Autodesk Inventor part; units mm, degrees
ref_plane "YZ Plane" through (0, 0, 0) normal (1, 0, 0) x (0, 1, 0)
ref_plane "XZ Plane" through (0, 0, 0) normal (0, 1, 0) x (-1, 0, 0)
ref_plane "XY Plane" through (0, 0, 0) normal (0, 0, 1) x (1, 0, 0)
sketch "Sketch1" plane through (0, 0, 0) normal (0, 1, 0) x (-1, 0, 0)
  line L0 (-45, 68.75) -> (45, 68.75)
  line L1 (45, 68.75) -> (45, -68.75)
  line L2 (45, -68.75) -> (-45, -68.75)
  line L3 (-45, -68.75) -> (-45, 68.75)
  line L4 (-45, 68.75) -> (45, -68.75) construction
  line L5 (45, 68.75) -> (-45, -68.75) construction
  point P0 (0, 0)
  dimension "d0" = 137.5
  dimension "d1" = 90
extrude "Extrusion1" add sketch "Sketch1" along normal blind 25
sketch "Sketch2" plane through (0, 25, 0) normal (0, 1, 0) x (1, 0, 0)
  line L0 (43.55, -67.3) -> (-43.55, -67.3)
  line L1 (-43.55, -67.3) -> (-43.55, 67.3)
  line L2 (-43.55, 67.3) -> (43.55, 67.3)
  line L3 (43.55, 67.3) -> (43.55, -67.3)
  line L4 (43.55, -67.3) -> (-43.55, 67.3) construction
  line L5 (-43.55, -67.3) -> (43.55, 67.3) construction
  point P0 (0, 0)
  dimension "d4" = 134.6
  dimension "d5" = 87.1
extrude "Extrusion2" cut sketch "Sketch2" against normal blind 23
sketch "Sketch4" plane through (0, 25, 0) normal (0, 1, 0) x (1, 0, 0)
  line L0 (-45, 68.75) -> (-45, -68.75)
  line L1 (-43.55, -67.3) -> (-43.55, 67.3)
  line L2 (-45, 59) -> (-43.55, 59)
  line L3 (-43.55, 59) -> (-43.55, 28.5)
  line L4 (-43.55, 28.5) -> (-45, 28.5)
  line L5 (-45, 28.5) -> (-45, 59)
  line L6 (41.75, -65.5) -> (-41.75, -65.5)
  line L7 (-41.75, -65.5) -> (-41.75, 65.5)
  line L8 (-41.75, 65.5) -> (41.75, 65.5)
  line L9 (41.75, 65.5) -> (41.75, -65.5)
  line L10 (41.75, -65.5) -> (-41.75, 65.5) construction
  line L11 (-41.75, -65.5) -> (41.75, 65.5) construction
  line L12 (-43.55, 67.3) -> (43.55, 67.3)
  line L13 (45, 68.75) -> (-45, 68.75)
  line L14 (17.25, 67.3) -> (27.25, 67.3)
  line L15 (27.25, 67.3) -> (27.25, 68.75)
  line L16 (27.25, 68.75) -> (17.25, 68.75)
  line L17 (17.25, 68.75) -> (17.25, 67.3)
  line L18 (43.55, 67.3) -> (43.55, -67.3)
  line L19 (45, -68.75) -> (45, 68.75)
  line L20 (43.55, 56) -> (45, 56)
  line L21 (45, 56) -> (45, 25.5)
  line L22 (45, 25.5) -> (43.55, 25.5)
  line L23 (43.55, 25.5) -> (43.55, 56)
  line L24 (43.55, -35.5) -> (45, -35.5)
  line L25 (45, -35.5) -> (45, -19.5)
  line L26 (45, -19.5) -> (43.55, -19.5)
  line L27 (43.55, -19.5) -> (43.55, -35.5)
  point P0 (0, 0)
  point P1 (45, 56)
  dimension "d10" = 30.5
  dimension "d11" = 131
  dimension "d12" = 83.5
  dimension "d13" = 6.5
  dimension "d16" = 10
  dimension "d17" = 14.5
  dimension "d18" = 30.5
  dimension "d19" = 9.5
  dimension "d20" = 30
  dimension "d21" = 16
extrude "Extrusion4" cut sketch "Sketch4" against normal blind 16 contours L2 L1 L4 L0 | L13 L15 L12 L17 | L19 L22 L18 L20 | L19 L24 L18 L26
sketch "Sketch5" plane through (0, 25, 0) normal (0, 1, 0) x (1, 0, 0)
  line L0 (41.75, -65.5) -> (-41.75, -65.5)
  line L1 (-41.75, -65.5) -> (-41.75, 65.5)
  line L2 (-41.75, 65.5) -> (41.75, 65.5)
  line L3 (41.75, 65.5) -> (41.75, -65.5)
  line L4 (41.75, -65.5) -> (-41.75, 65.5) construction
  line L5 (-41.75, -65.5) -> (41.75, 65.5) construction
  line L6 (43.55, 25.5) -> (43.55, -19.5)
  line L7 (45, -19.5) -> (45, 25.5)
  line L8 (43.55, -10) -> (45, -10)
  line L9 (45, -10) -> (45, 22.5)
  line L10 (45, 22.5) -> (43.55, 22.5)
  line L11 (43.55, 22.5) -> (43.55, -10)
  line L12 (-43.55, 67.3) -> (43.55, 67.3)
  line L13 (45, 68.75) -> (-45, 68.75)
  line L14 (-11.75, 67.3) -> (-24.75, 67.3)
  line L15 (-24.75, 67.3) -> (-24.75, 68.75)
  line L16 (-24.75, 68.75) -> (-11.75, 68.75)
  line L17 (-11.75, 68.75) -> (-11.75, 67.3)
  point P0 (0, 0)
  point P1 (43.55, 22.5)
  dimension "d26" = 131
  dimension "d27" = 83.5
  dimension "d28" = 55.5
  dimension "d29" = 32.5
  dimension "d43" = 13
  dimension "d44" = 17
extrude "Extrusion5" cut sketch "Sketch5" against normal blind 21 contours L10 L7 L8 L6 | L15 L13 L17 L12
sketch "Sketch6" plane through (0, 2, 0) normal (0, 1, 0) x (1, 0, 0)
  line L0 (41.75, -67.5) -> (-41.75, -67.5)
  line L1 (-41.75, -67.5) -> (-41.75, 67.5)
  line L2 (-41.75, 67.5) -> (41.75, 67.5)
  line L3 (41.75, 67.5) -> (41.75, -67.5)
  line L4 (41.75, -67.5) -> (-41.75, 67.5) construction
  line L5 (-41.75, -67.5) -> (41.75, 67.5) construction
  line L6 (-31.25, -53.5) -> (31.75, -53.5)
  line L7 (31.75, -53.5) -> (31.75, -34.5)
  line L8 (31.75, -34.5) -> (-31.25, -34.5)
  line L9 (-31.25, -34.5) -> (-31.25, -53.5)
  point P0 (0, 0)
  dimension "d32" = 135
  dimension "d33" = 83.5
  dimension "d34" = 19
  dimension "d35" = 63
  dimension "d36" = 10
  dimension "d37" = 14
extrude "Extrusion6" cut sketch "Sketch6" against normal through all contours L9 L8 L7 L6
fillet "Fillet1" radius 1.5 24 edges at (-43.55, 13.5, 67.3) (-43.55, 13.5, -67.3) (43.55, 13.5, -67.3) (43.55, 13.5, 67.3) (-31.25, 1, 34.5) (-31.25, 1, 53.5) (31.75, 1, 53.5) (31.75, 1, 34.5) (-44.275, 9, -28.5) (-44.275, 9, -59) (44.275, 9, 35.5) (44.275, 9, 19.5) (44.275, 4, 10) (44.275, 4, -22.5) (44.275, 9, -25.5) (44.275, 9, -56) (17.25, 9, -68.025) (27.25, 9, -68.025) (-45, 12.5, -68.75) (-45, 12.5, 68.75) (45, 12.5, 68.75) (45, 12.5, -68.75) (-11.75, 4, -68.025) (-24.75, 4, -68.025)
properties part number "BoardCover"
Could you check a few things on this model? Use its own coordinates, in mm. A direction names the side the tool comes from. Coordinates: 2 decimals unless noted, no trailing zeros. Order: outer loops, then holes, each group sorted by start corner. A loop starts at its lowest first (then second) coordinate and runs counter-clockwise, first axis right, second up. Notation, with made-up numbers: M 29,-27.5 L 71,-27.5 A29 cw 71,3.5 Z; hole C -14,-9 d8. An arc over 180 degrees is marked long. Use one line per item in the form item = value. Start each with the question number.
1. For pin 1 (1.2 mm diameter, centred on y = 20, z = -68, fed in from -X); pin 2 (1.6 mm diameter, centred on x = -44, y = 17, fed in from -Z); pin 3 (1.6 mm diameter, centred on x = 44.5, z = -10, fed in from +Y); pin 4 (0.7 mm diameter, centred on x = -44.5, z = -47, fed in from +Y), each with a flat end and sliding along its axis, tell me the tip position at first contact or that it passes through.
2. Please list where these lines run through material, in increasing order: line 1 (Z direction, x = -8, y = 14); line 2 (X direction, y = 6.75, z = 12); line 3 (Z direction, x = -30, y = 1.75).
3. Suppose I cut it at C-C on z = 31.5. Write out the boundary of the cut face in (x, y), then the cut area to 4 significant figures.
4. We'd pull the mould along X, two halves only. Please class faces 1 (the flat face through (1, 0, 1)), 2 (the flat face through (45, 10, 14)), 3 (the flat face through (-1, 2, -1)): +X half, -X half, draft (parallel to the pull), parting line (faces both ways), or undercut.
5. On a 3-axis mill with a long thin cutter (end or side, diameter ignored), from which of +Z, -Z, +X, -X, +Y, -Y can I reach the whole of each face in a straight line? I mean faces 4 (the flat face through (-1, 14, -67.3)), 5 (the flat face through (-37.1, 25, -67.5)). Say none if no direction works.
6. Suppose I cut it at D-D on x = 34.5. Write out the boundary of the cut face in (y, z).
7. Suppose I cut it at A-A on x = -19.5. Write out the boundary of the cut face in (y, z).
8. Suppose I cut it at B-B on z = 50.5. Write out the boundary of the cut face in (x, y).
Geometry says:
q1.pin_1 = -44.99
q1.pin_2 = -68.75
q1.pin_3 = 4
q1.pin_4 = 9
q2.line_1 = -68.75 to -67.3, 67.3 to 68.75
q2.line_2 = -45 to -43.55, 43.55 to 45
q2.line_3 = -68.75 to 34.52, 53.48 to 68.75
q3.outline = M -45,0 L 45,0 L 45,9 L 43.55,9 L 43.55,2 L -43.55,2 L -43.55,25 L -45,25 Z
q3.area = 223.5 mm^2
q4.face_1 = draft
q4.face_2 = +X half
q4.face_3 = undercut
q5.face_4 = +Y
q5.face_5 = +Z, -Z, +X, -X, +Y
q6.outline = M 0,-68.75 L 25,-68.75 L 25,-67.3 L 2,-67.3 L 2,67.3 L 25,67.3 L 25,68.75 L 0,68.75 Z
q7.outline = M 0,-68.75 L 4,-68.75 L 4,-67.3 L 2,-67.3 L 2,34.5 L 0,34.5 Z; M 0,53.5 L 2,53.5 L 2,67.3 L 25,67.3 L 25,68.75 L 0,68.75 Z
q8.outline = M -45,0 L -31.25,0 L -31.25,2 L -43.55,2 L -43.55,25 L -45,25 Z; M 31.75,0 L 45,0 L 45,25 L 43.55,25 L 43.55,2 L 31.75,2 Z
